The model under review builds one solid part; all positions refer to its coordinate system, in mm. Coordinates: 2 decimals unless noted, no trailing zeros. Order: outer loops, then holes, each group sorted by start corner. A loop starts at its lowest first (then second) coordinate and runs counter-clockwise, first axis right, second up. Notation, with made-up numbers: M 43,47 L 51,47 A16 cw 51,55 Z; hole C -30,75 d5. An arc over 180 degrees is marked long. One line per item, written item: value.
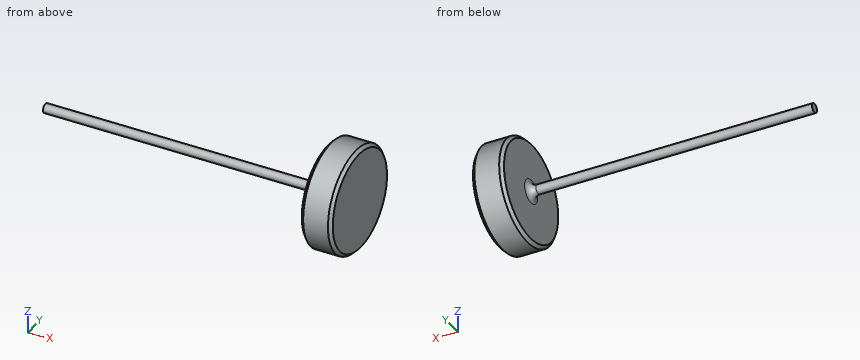
```python
from build123d import *

# Parameters (mm, degrees)
SKETCH1_R           = 31.75
BOSS_EXTRUDE1_DEPTH = 19.05
SKETCH2_R           = 2.794
BOSS_EXTRUDE2_DEPTH = 173.99
FILLET1_R           = 4.445
CHAMFER1_SIZE       = 1.905


with BuildPart() as part:
    # Sketch1 → Boss-Extrude1 (new body)
    with BuildSketch(Plane(origin=(0, 0, 0), x_dir=(0, 0, -1), z_dir=(1, 0, 0))):
        with Locations(Location((0, 0, 0), (0, 0, 180))):
            Circle(SKETCH1_R)
    extrude(amount=BOSS_EXTRUDE1_DEPTH)

    # Sketch2 → Boss-Extrude2 (add)
    with BuildSketch(Plane.ZY):
        with Locations(Location((0, 0, 0), (0, 0, 180))):
            Circle(SKETCH2_R)
    extrude(amount=BOSS_EXTRUDE2_DEPTH)

    # Fillet1
    fillet1_edges = [part.edges().sort_by_distance(p)[0] for p in [
        (0, 0, 2.794),
    ]]
    fillet(fillet1_edges, radius=FILLET1_R)

    # Chamfer1
    chamfer1_edges = [part.edges().sort_by_distance(p)[0] for p in [
        (0, 0, -31.75),
        (19.05, 0, -31.75),
    ]]
    chamfer(chamfer1_edges, length=CHAMFER1_SIZE)


solid = part.part
```
(1) For L1, parallel to X at y = 9, z = -18; L2, parallel to Y at x = 4, z = -21; L3, parallel to Y at x = -154, z = 1.5, list the stretches that pass through material, from the lowest coordinate up.
Geometry results:
L1: x = 0 to 19.05
L2: y = -23.81 to 23.81
L3: y = -2.36 to 2.36
(2) We need section A-A, the plane y = 0. State the section outline as (x, z) points (3 decimals).
Geometry results:
outline: M -173.99,-2.794 L -4.445,-2.794 A4.445 cw 0,-7.239 L 0,-29.845 L 1.905,-31.75 L 17.145,-31.75 L 19.05,-29.845 L 19.05,29.845 L 17.145,31.75 L 1.905,31.75 L 0,29.845 L 0,7.239 A4.445 cw -4.445,2.794 L -173.99,2.794 Z
(3) We need section C-C, the plane x = -50. State the section outline as (y, z) points, plus the area to 3 significant figures.
Geometry results:
outline: C 0,0 d5.59
area: 24.5 mm2
(4) Insertion check: pin 1 Ø12 at (x, z) = (-63, -6) entering from -Y; pin 2 Ø6 at (x, z) = (-91.5, -2) entering from +Y; pin 3 Ø12 at (y, z) = (-2, -4) entering from -X. Each pin has a flat end and moves straight along its axis. Give the tip position at first contact, or say it passes through.
Geometry results:
pin 1: stops at y = -2.79
pin 2: stops at y = 2.79
pin 3: stops at x = -173.99
